Design review of the part shown in the three views and the two pictorial views. Dimensions are in mm from the part's minimum x, y and z. Give positions to 0.01 mm unless a question says otherwise; leave off trailing zeros. Order: outer loops, then holes, each group sorted by start corner. A loop starts at its lowest first (then second) coordinate and runs counter-clockwise, first axis right, second up. Notation, with made-up numbers: M -36.5,16.25 L 4.5,16.25 A13 ccw 4.5,33.25 Z; hole C 58,-30.5 d8. An arc over 180 degrees is marked long. Answer as a JSON object with one key per item and string values.
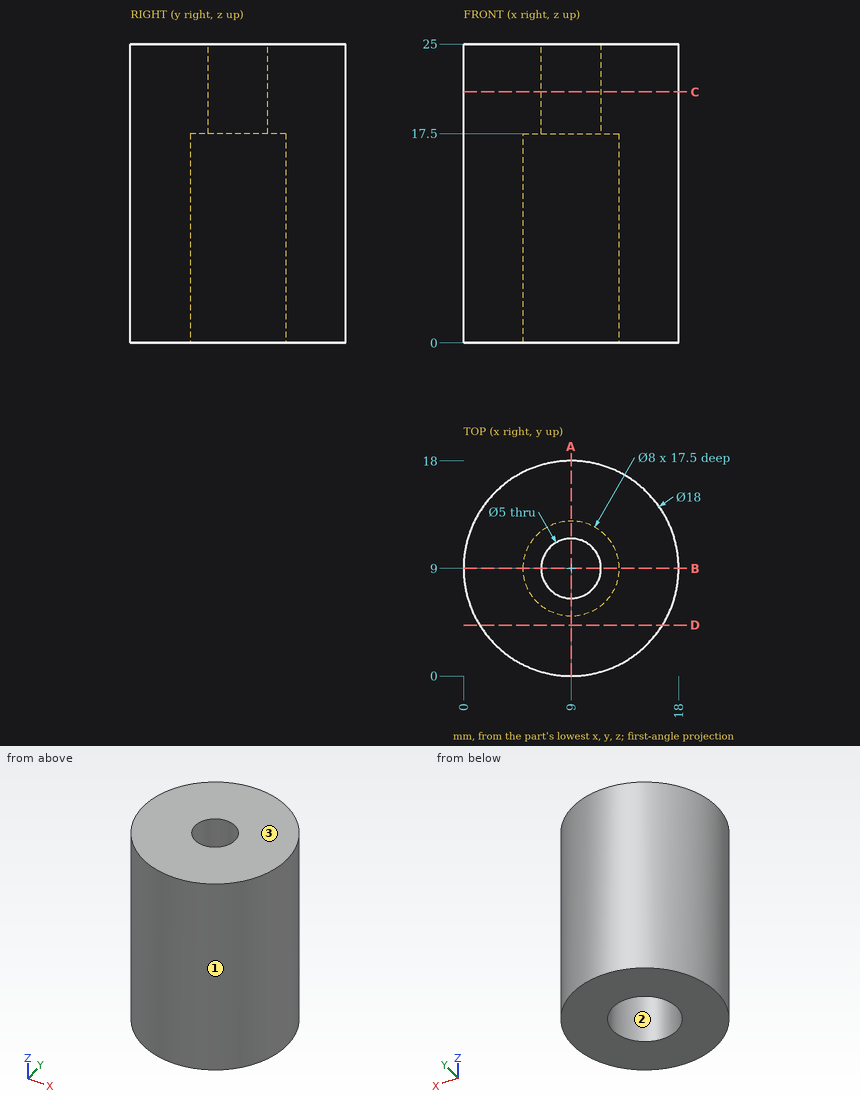
(1) We need section A-A (x = 9). Write out the cut boundary in (y, z).
Checked values:
{"outline": "M 0,0 L 5,0 L 5,17.5 L 6.5,17.5 L 6.5,25 L 0,25 Z; M 11.5,17.5 L 13,17.5 L 13,0 L 18,0 L 18,25 L 11.5,25 Z"}
(2) We need section C-C (z = 21). Write out the cut boundary in (x, y), plus the area to 3 significant figures.
Checked values:
{"outline": "C 9,9 d18; hole C 9,9 d5", "area": "235 mm^2"}
(3) Draft analysis for pull direction Y (two halves, no side actions). For the marked faces 1, 2 and 3, state which applies: +Y half, -Y half, draft (parallel to the pull), parting line (faces both ways), or undercut.
Checked values:
{"face 1": "parting line", "face 2": "undercut", "face 3": "draft"}
(4) We need section D-D (y = 4.25). Write out the cut boundary in (x, z), plus the area to 3 significant figures.
Checked values:
{"outline": "M 1.36,0 L 16.64,0 L 16.64,25 L 1.36,25 Z", "area": "382 mm^2"}
(5) To check wall thickness, follow L1, parallel to Y at x = 9, z = 9; L2, parallel to Z at x = 12.25, y = 8.5; L3, parallel to Y at x = 9.25, z = 18.25. State the ranges of each line that lie inside material, in increasing order. Write a range as from..to.
Checked values:
{"L1": "y = 0..5, 13..18", "L2": "z = 17.5..25", "L3": "y = 0..6.51, 11.49..18"}
(6) Insertion check: pin 1 (4 mm diameter, centred on x = 9, y = 10, fed in from -Z); pin 2 (8 mm diameter, centred on y = 3, z = 10, fed in from +X); pin 3 (7 mm diameter, centred on x = 9, y = 9, fed in from +Z); pin 4 (5 mm diameter, centred on y = 12.5, z = 4, fed in from +X). Each pin has a flat end and moves straight along its axis. Give the tip position at first contact, or say it passes through.
Checked values:
{"pin 1": "stops at z = 17.5", "pin 2": "stops at x = 17.77", "pin 3": "stops at z = 25", "pin 4": "stops at x = 17.94"}
